For this review, take the finished solid that the model builds, in its own axes (mm). A direction names the side the tool comes from. Coordinates: 2 decimals unless noted, no trailing zeros. Order: outer loops, then holes, each group sorted by start corner. A loop starts at its lowest first (then second) coordinate and runs counter-clockwise, first axis right, second up. Notation, with made-up numbers: (47.5, -5) -> (51.5, -5) arc R23 cw to (51.5, 6) -> close; hole circle Ø11 at (78, 24.5). An arc over 180 degrees is marked (long way). Answer as a JSON object with one key per item and string values. Group by question number.
1) Add section D-D, the plane x = 27. Write out the cut boundary in (y, z), then the cut area to 3 significant figures.
2) Add section A-A, the plane y = 43.5. Write out the cut boundary in (x, z).
3) Add section B-B, the plane x = -118. Write out the cut boundary in (y, z).
4) Draft analysis for pull direction Y (two halves, no side actions). For faces 1 (the flat face through (-3, -101.6, 100)), 2 (the flat face through (203.2, -89, 100)), 3 (the flat face through (-12.7, -1, 100)), state which applies: +Y half, -Y half, draft (parallel to the pull), parting line (faces both ways), or undercut.
5) Add section C-C, the plane z = 16. Count the separate pieces of the cut face and the enclosed holes in it, then the cut area to 3 significant figures.
6) Machinability: for faces 4 (the flat face through (-90, 76.2, 100)), 5 (the flat face through (190.5, -1, 100)), 6 (the flat face through (-190.5, 1, 100)), which of the approach directions +Z, -Z, +X, -X, +Y, -Y give a long, thin tool a straight path to every point of the face, cutting with its end or side? Answer none if there is none.
7) Wall thickness on L1, parallel to X at y = -21, z = 145; L2, parallel to Y at x = -122, z = 31; L3, parallel to X at y = 71.5, z = 82.5: over which ranges is each line inside the solid? List them lowest first.
8) For pin 1 (1 mm diameter, centred on y = 60.5, z = 173.5, fed in from -X); pin 2 (8 mm diameter, centred on x = 160, y = -12.5, fed in from +Z), all flat-tipped, find the tip position at first contact; note any pin that passes through.
from build123d import *

# Parameters (mm, degrees)
F0_W     = 152.4
F0_H     = 152.4
F1_DEPTH = 203.2
F2_R     = 25.4
F3_R     = 5


with BuildPart() as f1:
    # F0 (on Top) → F1 (new body)
    with BuildSketch(Plane.XY):
        Polygon((203.2, 101.6), (-203.2, 101.6), (-203.2, 76.2), (-190.5, 76.2), (-190.5, -76.2), (-203.2, -76.2), (-203.2, -101.6), (203.2, -101.6), (203.2, -76.2), (190.5, -76.2), (190.5, 76.2), (203.2, 76.2), align=None)
        with Locations((-88.9, 0)):
            Rectangle(F0_W, F0_H, mode=Mode.SUBTRACT)
        with Locations((88.9, 0)):
            Rectangle(F0_W, F0_H, mode=Mode.SUBTRACT)
    extrude(amount=F1_DEPTH)

    # F2
    f2_edges = [f1.edges().sort_by_distance(p)[0] for p in [
        (-165.1, 76.2, 101.6),
        (-165.1, -76.2, 101.6),
        (12.7, -76.2, 101.6),
        (12.7, 76.2, 101.6),
        (165.1, 76.2, 101.6),
        (165.1, -76.2, 101.6),
        (-12.7, 76.2, 101.6),
        (-12.7, -76.2, 101.6),
    ]]
    fillet(f2_edges, radius=F2_R)

    # F3
    f3_edges = [f1.edges().sort_by_distance(p)[0] for p in [
        (-190.5, 76.2, 101.6),
        (-190.5, -76.2, 101.6),
        (190.5, 76.2, 101.6),
        (190.5, -76.2, 101.6),
    ]]
    fillet(f3_edges, radius=F3_R)


solid = f1.part
Output values:
{
 "1": {"outline": "(-101.6, 0) -> (-73.65, 0) -> (-73.65, 203.2) -> (-101.6, 203.2) -> close; (73.65, 0) -> (101.6, 0) -> (101.6, 203.2) -> (73.65, 203.2) -> close", "area": "11,400 mm²"},
 "2": {"outline": "(-190.5, 0) -> (-165.1, 0) -> (-165.1, 203.2) -> (-190.5, 203.2) -> close; (-12.7, 0) -> (12.7, 0) -> (12.7, 203.2) -> (-12.7, 203.2) -> close; (165.1, 0) -> (190.5, 0) -> (190.5, 203.2) -> (165.1, 203.2) -> close"},
 "3": {"outline": "(-101.6, 0) -> (-76.2, 0) -> (-76.2, 203.2) -> (-101.6, 203.2) -> close; (76.2, 0) -> (101.6, 0) -> (101.6, 203.2) -> (76.2, 203.2) -> close"},
 "4": {"face 1": "-Y half", "face 2": "draft", "face 3": "undercut"},
 "5": {"separate pieces": "1", "enclosed holes": "2", "area": "33,400 mm²"},
 "6": {"face 4": "+Z, -Z", "face 5": "+Z, -Z, +X", "face 6": "+Z, -Z, -X"},
 "7": {"L1": "x = -190.5 to -165.1, -12.7 to 12.7, 165.1 to 190.5", "L2": "y = -101.6 to -76.2, 76.2 to 101.6", "L3": "x = -190.51 to -154.42, -23.38 to 23.38, 154.42 to 190.51"},
 "8": {"pin 1": "stops at x = -190.5", "pin 2": "passes through"}
}
